from build123d import *

# Parameters (mm, degrees)
BORESKETCH_R       = 50.8
BORE_DEPTH         = 75.676
SKETCH3_R          = 9.525
BOLT_HOLE_DEPTH    = 69.326
BOLT_PATTERN_COUNT = 8


with BuildPart() as part:
    # Main → Revolve1 (revolve)
    with BuildSketch(Plane.XY):
        Polygon((0, 0), (-78.613, 0), (-78.613, -6.35), (-114.3, -6.35), (-114.3, -30.226), (-67.437, -30.226), (-57.15, -66.378666667), (-57.15, -74.676), (0, -74.676), align=None)
    revolve(axis=Axis((0, 0, 0), (0, -1, 0)))

    # BoreSketch → Bore (cut, through all)
    with BuildSketch(Plane(origin=(0, 0, 0), x_dir=(1, 0, 0), z_dir=(0, 1, 0))):
        Circle(BORESKETCH_R)
    extrude(amount=-BORE_DEPTH, mode=Mode.SUBTRACT)

    # Sketch3 → Bolt Hole (cut, through all)
    with BuildSketch(Plane(origin=(0, -6.35, 0), x_dir=(1, 0, 0), z_dir=(0, 1, 0))):
        with Locations((-36.450596933, 87.999525472)):
            Circle(SKETCH3_R)
    bolt_hole = extrude(amount=-BOLT_HOLE_DEPTH, mode=Mode.SUBTRACT)

    # Bolt Pattern: Bolt Hole ×8 about axis
    bolt_pattern_axis = Axis((0, 0, 0), (0, 1, 0))
    for i in range(1, BOLT_PATTERN_COUNT):
        add(bolt_hole.rotate(bolt_pattern_axis, i * 360 / BOLT_PATTERN_COUNT), mode=Mode.SUBTRACT)


solid = part.part
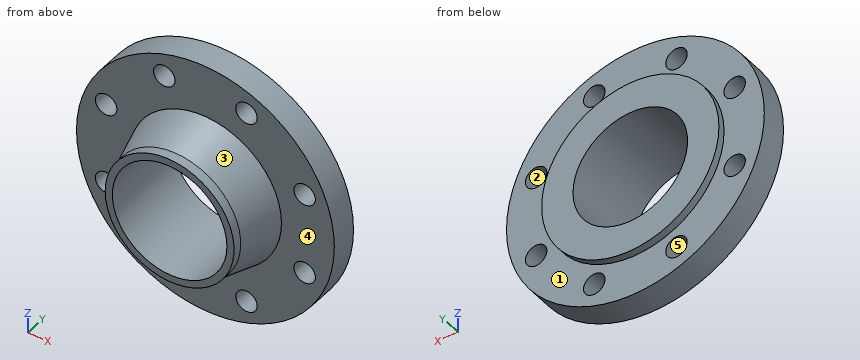
Can you work these out from the model? Positions are in its coordinate system, mm. Face numbers are marked on the shaded views. A direction names the side the tool comes from. Round coordinates to 2 decimals unless told otherwise and drop trailing zeros. Write each loop counter-clockwise with the first axis right and the second up, starting at its lowest first coordinate (ties: lowest second). Pieces come first, ordered by that corner, then holes. Notation, with made-up numbers: (-20.5, -25.5) -> (17.5, -25.5) arc R23 ccw to (17.5, 1.5) -> close; hole circle Ø4 at (-23.5, 63.5). An arc over 180 degrees is marked (long way). Use one line per item in the form item = value. Start each with the question number.
Q1. Imagine slicing it at A-A (x = 0). Please give me the cut outline in (y, z).
Q2. If I drill on probe 1 along X at (y, z) = (-25, 0); probe 2 along Z at (x, y) = (-38, -12.5); probe 3 along X at (y, z) = (-17, -88.5), over which ranges is the centre line in solid material (lowest first)? Write a range as [from, to].
Q3. We'd pull the mould along X, two halves only. Please class the marked faces 3, 4 and 5: +X half, -X half, draft (parallel to the pull), parting line (faces both ways), or undercut.
Q4. Imagine slicing it at B-B (z = 0). Please give me the cut outline in (x, y), then the cut area to 3 significant figures.
Q5. I'm going to push flat-ended pins straight in: P1, Ø25, axis at x = -88, z = -36.45, coming from the -Y side; P2, Ø4, axis at x = 75.5, y = -18, coming from the -Z side; P3, Ø4, axis at y = -57, z = 40, coming from the +X side; P4, Ø12, axis at x = -1.5, z = -67, coming from the +Y side. Where does each tip first touch, or does it pass through?
Q6. Which directions (+Z, -Z, +X, -X, +Y, -Y) give clear straight access to the entire face, cutting with the end or side of a thin tool? Please do the marked faces 1 and 2.
Q7. Imagine slicing it at C-C (y = -25). Count the separate pieces of the cut face and the enclosed holes in it, then the cut area to 3 significant figures.
Worked out:
q1.outline = (-74.68, -57.15) -> (-66.38, -57.15) -> (-30.23, -67.44) -> (-30.23, -114.3) -> (-6.35, -114.3) -> (-6.35, -78.61) -> (0, -78.61) -> (0, -50.8) -> (-74.68, -50.8) -> close; (-74.68, 50.8) -> (0, 50.8) -> (0, 78.61) -> (-6.35, 78.61) -> (-6.35, 114.3) -> (-30.23, 114.3) -> (-30.23, 67.44) -> (-66.38, 57.15) -> (-74.68, 57.15) -> close
q2.probe_1 = [-114.3, -50.8], [50.8, 114.3]
q2.probe_2 = [-107.8, -97.4], [-78.6, -33.71], [33.71, 78.6], [97.4, 107.8]
q2.probe_3 = [-72.33, -45.96], [-26.94, 26.94], [45.96, 72.33]
q3.face_3 = parting line
q3.face_4 = draft
q3.face_5 = undercut
q4.outline = (-114.3, -30.23) -> (-67.44, -30.23) -> (-57.15, -66.38) -> (-57.15, -74.68) -> (-50.8, -74.68) -> (-50.8, 0) -> (-78.61, 0) -> (-78.61, -6.35) -> (-114.3, -6.35) -> close; (50.8, -74.68) -> (57.15, -74.68) -> (57.15, -66.38) -> (67.44, -30.23) -> (114.3, -30.23) -> (114.3, -6.35) -> (78.61, -6.35) -> (78.61, 0) -> (50.8, 0) -> close
q4.area = 4,320 mm^2
q5.P1 = -30.23
q5.P2 = -87.53
q5.P3 = 46.36
q5.P4 = 0
q6.face_1 = +Y
q6.face_2 = +Y, -Y
q7.separate_pieces = 1
q7.enclosed_holes = 9
q7.area = 30,700 mm^2
